Could you check a few things on this drawing? It's one solid part, dimensions in mm from its lowest x, y, z. A direction names the side the tool comes from. Give positions to 0.01 mm unless a question says otherwise; leave off trailing zeros. Order: outer loops, then holes, each group sorted by start corner. A loop starts at its lowest first (then second) coordinate and runs counter-clockwise, first axis right, second up. Notation, with made-up numbers: M 54.5,85.5 L 78.5,85.5 A36 cw 78.5,122.5 Z; hole C 32.5,70.5 d7. An arc over 180 degrees is marked long. Use one line per item in the form item = value.
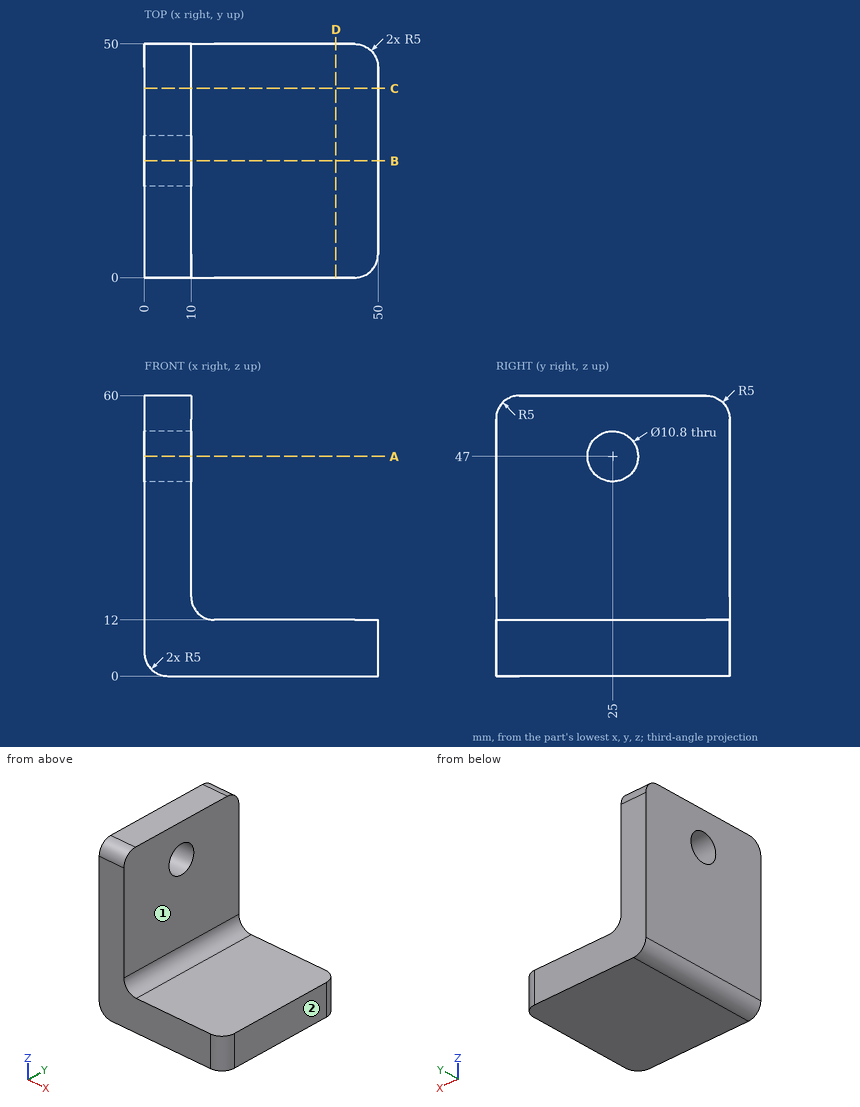
Q1. On a 3-axis mill with a long thin cutter (end or side, diameter ignored), from which of +Z, -Z, +X, -X, +Y, -Y can I reach the whole of each face in a straight line? I mean the marked faces 1 and 2. Say none if no direction works.
Found:
face_1 = +Z, +X, +Y, -Y
face_2 = +Z, -Z, +X, +Y, -Y
Q2. I want a section at C-C on y = 40.5. Write out the boundary of the cut face in (x, z).
Found:
outline = M 0,5 A5 ccw 5,0 L 50,0 L 50,12 L 15,12 A5 cw 10,17 L 10,60 L 0,60 Z
Q3. I want a section at B-B on y = 25. Write out the boundary of the cut face in (x, z).
Found:
outline = M 0,5 A5 ccw 5,0 L 50,0 L 50,12 L 15,12 A5 cw 10,17 L 10,41.6 L 0,41.6 Z; M 0,52.4 L 10,52.4 L 10,60 L 0,60 Z
Q4. I want a section at A-A on z = 47. Write out the boundary of the cut face in (x, y), then the cut area to 3 significant figures.
Found:
outline = M 0,0 L 10,0 L 10,19.6 L 0,19.6 Z; M 0,30.4 L 10,30.4 L 10,50 L 0,50 Z
area = 392 mm²
Q5. I want a section at D-D on x = 41. Write out the boundary of the cut face in (y, z), then the cut area to 3 significant figures.
Found:
outline = M 0,0 L 50,0 L 50,12 L 0,12 Z
area = 600 mm²
Q6. I'm going to push flat-ended pins straight in: pin 1 Ø21.5 at (y, z) = (35.5, 32.5) entering from +X; pin 2 Ø6 at (y, z) = (44, 17.5) entering from +X; pin 3 Ø10.5 at (x, y) = (32.5, 23) entering from +Z. Where does each tip first touch, or does it pass through?
Found:
pin_1 = 10
pin_2 = 10.67
pin_3 = 12
Q7. I need wall thicknesses on L1, parallel to Z at x = 4.75, y = 25; L2, parallel to Z at x = 15, y = 15; L3, parallel to X at y = 32.5, z = 47.5. Which ranges of each line are inside material? Lowest first, please.
Found:
L1 = 0.01 to 41.6, 52.4 to 60
L2 = 0 to 12
L3 = 0 to 10
